Verification items for the finished model (mm, model axes). A direction names the side the tool comes from. Coordinates: 2 decimals unless noted, no trailing zeros. Order: outer loops, then holes, each group sorted by start corner. A loop starts at its lowest first (then second) coordinate and runs counter-clockwise, first axis right, second up. Notation, with made-up numbers: M 77,68.25 L 118,68.25 A11 ccw 118,84.25 Z; hole C 83.25,-11.5 d11. An arc over 180 degrees is marked long. Return JSON: item names as keys, results as strings.
Autodesk Inventor part; units mm, degrees
ref_plane "YZ Plane" through (0, 0, 0) normal (1, 0, 0) x (0, 1, 0)
ref_plane "XZ Plane" through (0, 0, 0) normal (0, 1, 0) x (-1, 0, 0)
ref_plane "XY Plane" through (0, 0, 0) normal (0, 0, 1) x (1, 0, 0)
sketch "スケッチ1" plane through (0, 0, 0) normal (0, 0, 1) x (1, 0, 0)
  arc A0 (-2.6047, -14.7721) -> (15, 0) centre (0, 0) ccw construction
  arc A1 (-2.0751, -11.7685) -> (11.5542, -3.05) centre (0, 0) ccw
  arc A2 (-2.0751, -11.7685) -> (-2.602, -11.7221) centre (-2.6047, -14.7721) ccw
  line L0 (0, 0) -> (-6, 0) construction
  line L1 (0, 3.05) -> (-6, 3.05)
  line L2 (-6, -3.05) -> (0, -3.05)
  arc A3 (0, -3.05) -> (0, 3.05) centre (0, 0) ccw
  arc A4 (-6, 3.05) -> (-6, -3.05) centre (-6, 0) ccw
  line L3 (15, 0) -> (9, 0) construction
  line L4 (15, 3.05) -> (9, 3.05)
  arc A5 (9, 3.05) -> (9, -3.05) centre (9, 0) ccw
  line L5 (-161, 7.05) -> (9, 7.05)
  line L6 (-161, 7.05) -> (-143.3628, -2.95)
  line L7 (-2.602, -11.7221) -> (-143.3628, -2.95)
  arc A6 (17.9444, -0.7957) -> (15, 3.05) centre (15, 0) ccw
  line L8 (9, -3.05) -> (11.5542, -3.05)
  line L9 (14.6866, -3.05) -> (14.3582, -3.05)
  circle A7 centre (21.3232, -1.7088) radius 1.5
  arc A8 (17.9444, -0.7957) -> (23.4882, 1.0412) centre (21.3232, -1.7088) ccw
  line L10 (9, 7.05) -> (15.8557, 7.05)
  line L11 (15.8557, 7.05) -> (23.4882, 1.0412)
  point P0 (-3, 0)
  point P1 (12, 0)
  dimension "d0" = 15
  dimension "d1" = 6.1
  dimension "d2" = 6
  dimension "d3" = 6.1
  dimension "d4" = 6
  dimension "d5" = 6.1
  dimension "d6" = 100
  dimension "d8" = 4
  dimension "d9" = 10
  dimension "d17" = 3
  dimension "d19" = 2
  dimension "d20" = 170
extrude "押し出し1" add sketch "スケッチ1" along normal blind 5
fillet "フィレット1" radius 2 2 edges at (-161, 7.05, 2.5) (-143.3628, -2.95, 2.5)
fillet "フィレット3" radius 1 1 edges at (11.5542, -3.05, 2.5)
properties part number "ウイング仮" material "ポリカーボネート、クリア"
Q1. Draft check along X on faces 3 (the face through (17.398, 1.885, 2.465)), 4 (the face through (19.6, 4.1, 2.5)), 5 (the face through (-67, 0, 0)). Enter one of: pulls with the +X half, pulls with the -X half, needs draft (parallel to the pull), parting line crosses it, or undercut.
Values:
{"face 3": "undercut", "face 4": "pulls with the +X half", "face 5": "needs draft"}
Q2. Cross-section at A-A, the plane z = 1. Record the boundary of the cut face in (x, y), and give its area (3 significant figures).
Values:
{"outline": "M -154.4,3.31 L -143.76,-2.72 A2 ccw -142.9,-2.98 L -2.6,-11.72 A3.06 cw -2.08,-11.77 A11.95 ccw 11.1,-4.42 A1 ccw 10.17,-3.05 L 9,-3.05 A3.05 cw 9,3.05 L 15,3.05 A3.05 cw 17.94,-0.8 A3.5 ccw long 23.49,1.04 L 15.86,7.05 L -153.42,7.05 A2 ccw Z; hole M -6,-3.05 L 0,-3.05 A3.05 ccw 0,3.05 L -6,3.05 A3.05 ccw Z; hole C 21.32,-1.71 d3", "area": "2,320 mm^2"}
Q3. Material ranges on line 1 along X through (y, z) = (2, 0.6); line 2 along Y through (x, z) = (0, 1.2); line 3 along Y through (x, z) = (8.5, 1.4), recorded low to high.
Values:
{"line 1": "-152.09 to -8.3, 2.3 to 6.7, 17.3 to 22.27", "line 2": "-11.95 to -3.05, 3.05 to 7.05", "line 3": "-8.4 to -3.01, 3.01 to 7.05"}
Q4. Cross-section at C-C, the plane x = -46. Record the boundary of the cut face in (y, z), and give its area (3 significant figures).
Values:
{"outline": "M -9.02,0 L 7.05,0 L 7.05,5 L -9.02,5 Z", "area": "80.3 mm^2"}
Q5. Tool access check on faces 1 (the face through (-155.34, 5.6, 2.54)), 2 (the face through (-3, 3.05, 2)). Record the directions out of +Z, -Z, +X, -X, +Y, -Y that give a thin tool (end or side, any length) a straight path to the whole face; none if there is none.
Values:
{"face 1": "+Z, -Z, -X", "face 2": "+Z, -Z"}
Q6. Cross-section at B-B, the plane y = -7. Record the boundary of the cut face in (x, z).
Values:
{"outline": "M -78.37,0 L 9.69,0 L 9.69,5 L -78.37,5 Z"}
Q7. Go/stop test with flat-tipped pins: pin 1 (3 mm diameter, centred on x = -74.5, z = 2, fed in from -Y); pin 2 (3 mm diameter, centred on x = -131, z = 1, fed in from -Y); pin 3 (2.5 mm diameter, centred on x = -4, z = 3, fed in from -Y). Record where each tip stops, or that it passes through.
Values:
{"pin 1": "y = -7.33", "pin 2": "y = -3.81", "pin 3": "y = -11.71"}
